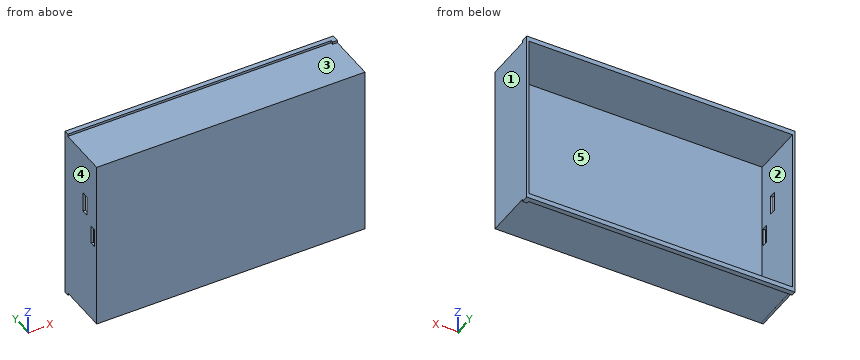
from build123d import *

# Parameters (mm, degrees)
CROQUIS1_W              = 112
CROQUIS1_H              = 72
SALIENTE_EXTRUIR1_DEPTH = 1
SALIENTE_EXTRUIR2_DEPTH = 1
CROQUIS3_W              = 72
CROQUIS3_H              = 23
SALIENTE_EXTRUIR3_DEPTH = 1
CROQUIS4_W              = 112
CROQUIS4_H              = 23
SALIENTE_EXTRUIR4_DEPTH = 1
CROQUIS5_W              = 112
CROQUIS5_H              = 23
SALIENTE_EXTRUIR5_DEPTH = 1
CROQUIS6_W              = 7.7
CROQUIS6_H              = 2.5
CROQUIS6_W_2            = 8.3
CROQUIS6_H_2            = 3
CORTAR_EXTRUIR1_DEPTH   = 1
SALIENTE_EXTRUIR6_DEPTH = 1
SALIENTE_EXTRUIR7_DEPTH = 1


with BuildPart() as part:
    # Croquis1 → Saliente-Extruir1 (new body)
    with BuildSketch(Plane(origin=(0, 0, 0), x_dir=(1, 0, 0), z_dir=(0, 1, 0))):
        with Locations((56, 36)):
            Rectangle(CROQUIS1_W, CROQUIS1_H)
    extrude(amount=SALIENTE_EXTRUIR1_DEPTH)

    # Croquis2 → Saliente-Extruir2 (add)
    with BuildSketch(Plane.ZY):
        Polygon((0, 0), (0, 23), (-72.007399111, 23), (-72, 0), align=None)
    extrude(amount=-SALIENTE_EXTRUIR2_DEPTH)

    # Croquis3 → Saliente-Extruir3 (add)
    with BuildSketch(Plane(origin=(112, 0, 0), x_dir=(0, 0, -1), z_dir=(1, 0, 0))):
        with Locations((36, 11.5)):
            Rectangle(CROQUIS3_W, CROQUIS3_H)
    extrude(amount=-SALIENTE_EXTRUIR3_DEPTH)

    # Croquis4 → Saliente-Extruir4 (add)
    with BuildSketch(Plane.XY):
        with Locations((56, 11.5)):
            Rectangle(CROQUIS4_W, CROQUIS4_H)
    extrude(amount=-SALIENTE_EXTRUIR4_DEPTH)

    # Croquis5 → Saliente-Extruir5 (add)
    with BuildSketch(Plane(origin=(0, 0, -72), x_dir=(-1, 0, 0), z_dir=(0, 0, -1))):
        with Locations((-56, 11.5)):
            Rectangle(CROQUIS5_W, CROQUIS5_H)
    extrude(amount=-SALIENTE_EXTRUIR5_DEPTH)

    # Croquis6 → Cortar-Extruir1 (cut)
    with BuildSketch(Plane.ZY):
        with Locations((-33.65, 2.75)):
            Rectangle(CROQUIS6_W, CROQUIS6_H)
        with Locations((-22.65, 8.5)):
            Rectangle(CROQUIS6_W_2, CROQUIS6_H_2)
    extrude(amount=-CORTAR_EXTRUIR1_DEPTH, mode=Mode.SUBTRACT)

    # Croquis7 → Saliente-Extruir6 (add)
    with BuildSketch(Plane(origin=(0, 0, -72), x_dir=(-1, 0, 0), z_dir=(0, 0, -1))):
        Polygon((-112, 23), (0, 23), (0, 21), (-110, 21), (-110, 20), (-112, 20), align=None)
    extrude(amount=SALIENTE_EXTRUIR6_DEPTH)

    # Croquis8 → Saliente-Extruir7 (add)
    with BuildSketch(Plane.XY):
        Polygon((112, 23), (112, 20), (110, 20), (110, 21), (0, 21), (0, 23), align=None)
    extrude(amount=SALIENTE_EXTRUIR7_DEPTH)


solid = part.part
Build history of the part. All positions in model axes, mm. Face numbers are marked on the shaded views. A direction names the side the tool comes from. Coordinates: 2 decimals unless noted, no trailing zeros. Write each loop counter-clockwise with the first axis right and the second up, starting at its lowest first coordinate (ties: lowest second). Pieces come first, ordered by that corner, then holes.
(1) Drill centre lines: line 1 (X direction, y = 8.5, z = -43); line 2 (Z direction, x = 37.5, y = 18); line 3 (Y direction, x = 79.5, z = -27.5). Where is each one in solid material? Low to high.
(2) 3-axis set-ups, long thin cutter, end or side, ignore diameter. For the marked faces 4 and 5: which of +Z, -Z, +X, -X, +Y, -Y reach the whole face in a straight line?
(3) Mould opens along X. For the marked faces 1, 2 and 3 say: pulls with the +X half, pulls with the -X half, needs draft (parallel to the pull), parting line crosses it, or undercut.
(4) Cut at A-A on z = -21. List the corners of the cut face in (x, y).
(5) Cut at B-B on x = 71.5. List the corners of the cut face in (y, z), and give its area (3 significant figures).
(6) Pin check, flat tips, straight feed: pin 1 Ø4 at (x, y) = (95, 5.5) entering from +Z; pin 2 Ø0.5 at (y, z) = (20.5, 0.5) entering from -X; pin 3 Ø4 at (x, z) = (61.5, -39) entering from +Y. Stop position of each tip, or through.
Working result:
1. line 1: x = 0 to 1, 111 to 112
1. line 2: z = -72 to -71, -1 to 0
1. line 3: y = 0 to 1
2. face 4: +Z, -Z, -X, +Y, -Y
2. face 5: +Y
3. face 1: pulls with the +X half
3. face 2: undercut
3. face 3: needs draft
4. outline: (0, 0) - (112, 0) - (112, 23) - (111, 23) - (111, 1) - (1, 1) - (1, 7) - (0, 7) - close; (0, 10) - (1, 10) - (1, 23) - (0, 23) - close
5. outline: (0, -72) - (21, -72) - (21, -73) - (23, -73) - (23, -71) - (1, -71) - (1, -1) - (23, -1) - (23, 1) - (21, 1) - (21, 0) - (0, 0) - close
5. area: 120 mm2
6. pin 1: stops at z = 0
6. pin 2: stops at x = 110
6. pin 3: stops at y = 1
